```python
from build123d import *

# Parameters (mm, degrees)
BOSS_EXTRUDE1_DEPTH = 1


with BuildPart() as part:
    # Sketch1 → Revolve1 (revolve)
    with BuildSketch(Plane(origin=(0, 0, 0), x_dir=(1, 0, 0), z_dir=(0, 1, 0))):
        Polygon((0, 15.606821862), (12, 15.606821862), (12, -8.393178138), (9.5, -8.393178138), (9.5, -11.393178138), (1, -11.393178138), (1, -19.393178138), (0, -19.393178138), align=None)
    revolve(axis=Axis((0, 0, 19.393178138), (0, 0, -1)))

    # Sketch3 → Boss-Extrude1 (add, symmetric)
    with BuildSketch(Plane(origin=(0, 0, 0), x_dir=(1, 0, 0), z_dir=(0, 1, 0))):
        with BuildLine():
            Line((9.289467417, 15.291250115), (7.355842044, 18.774923355))
            ThreePointArc((7.355842044, 18.774923355), (7.60881313, 19.659037934), (8.492927709, 19.406066848))
            Line((8.492927709, 19.406066848), (10.426553083, 15.922393608))
            ThreePointArc((10.426553083, 15.922393608), (10.173581996, 15.038279029), (9.289467417, 15.291250115))
        make_face()
        with BuildLine():
            Line((-9.289467417, 15.291250115), (-7.355842044, 18.774923355))
            ThreePointArc((-7.355842044, 18.774923355), (-7.60881313, 19.659037934), (-8.492927709, 19.406066848))
            Line((-8.492927709, 19.406066848), (-10.426553083, 15.922393608))
            ThreePointArc((-10.426553083, 15.922393608), (-10.173581996, 15.038279029), (-9.289467417, 15.291250115))
        make_face()
    extrude(amount=BOSS_EXTRUDE1_DEPTH, both=True)


solid = part.part
```
Verification items for the finished model (mm, model axes). A direction names the side the tool comes from. Coordinates: 2 decimals unless noted, no trailing zeros. Loops run counter-clockwise (first coordinate to the right, second up) from the corner with the lowest first, then second, coordinate; pieces in that order, holes last. Notation, with made-up numbers: (78.25, 16) - (129.25, 16) arc R21 cw to (129.25, 50) - close; hole circle Ø11 at (-28.5, -8.75). An arc over 180 degrees is marked (long way). Answer as a JSON object with one key per item and string values.
(1) Cross-section at D-D, the plane y = -5.75. Record the boundary of the cut face in (x, z).
Response:
{"outline": "(-10.53, -15.61) - (10.53, -15.61) - (10.53, 8.39) - (7.56, 8.39) - (7.56, 11.39) - (-7.56, 11.39) - (-7.56, 8.39) - (-10.53, 8.39) - close"}
(2) Cross-section at C-C, the plane z = 13.5. Record the boundary of the cut face in (x, y), then the cut area to 3 significant figures.
Response:
{"outline": "circle Ø2 at (0, 0)", "area": "3.14 mm²"}
(3) Cross-section at B-B, the plane x = 0. Record the boundary of the cut face in (y, z), then the cut area to 3 significant figures.
Response:
{"outline": "(-12, -15.61) - (12, -15.61) - (12, 8.39) - (9.5, 8.39) - (9.5, 11.39) - (1, 11.39) - (1, 19.39) - (-1, 19.39) - (-1, 11.39) - (-9.5, 11.39) - (-9.5, 8.39) - (-12, 8.39) - close", "area": "649 mm²"}
(4) Access from +Z, -Z, +X, -X, +Y, -Y to the whole of each face (thin tool, end or side, straight path). Record for faces 1 (the flat face through (-9.446, 0.014, -17.689)), 2 (the flat face through (8.247, -0.014, -17.169)), 3 (the flat face through (-9, -1, -18)), 4 (the flat face through (-9, 1, -18)), 5 (the flat face through (9, -4, 8.393)).
Response:
{"face 1": "-Z, -X, +Y, -Y", "face 2": "+Y, -Y", "face 3": "-Z, +X, -X, -Y", "face 4": "-Z, +X, -X, +Y", "face 5": "+Z"}
(5) Go/stop test with flat-tipped pins: pin 1 Ø1.5 at (x, y) = (-2, -8.5) entering from -Z; pin 2 Ø1 at (y, z) = (-1, -14) entering from +X; pin 3 Ø6 at (y, z) = (0.5, -4.5) entering from -X; pin 4 Ø1.6 at (x, z) = (9.5, -18) entering from +Y. Record where each tip stops, or that it passes through.
Response:
{"pin 1": "stops at z = -15.61", "pin 2": "stops at x = 11.99", "pin 3": "stops at x = -12", "pin 4": "stops at y = 1"}
(6) Mould release check, pull along X, two halves, no side actions. Record for faces 6 (the flat face through (-8.247, 0.014, -17.169)), 7 (the flat face through (9, -1, -18)), 8 (the flat face through (9.446, -0.014, -17.689)): pulls with the +X half, pulls with the -X half, needs draft (parallel to the pull), parting line crosses it, or undercut.
Response:
{"face 6": "undercut", "face 7": "needs draft", "face 8": "pulls with the +X half"}
(7) Scan lines: line 1 along Z through (x, y) = (3.5, 8.5); line 2 along Z through (x, y) = (-1.5, -10); line 3 along Y through (x, z) = (6.25, 0). Record each from-to range of solid material in increasing order.
Response:
{"line 1": "z = -15.61 to 11.39", "line 2": "z = -15.61 to 8.39", "line 3": "y = -10.24 to 10.24"}
(8) Cross-section at A-A, the plane y = 0. Record the boundary of the cut face in (x, z).
Response:
{"outline": "(-12, -15.61) - (-10.51, -15.61) arc R0.65 ccw to (-10.43, -15.92) - (-8.49, -19.41) arc R0.65 ccw to (-7.36, -18.77) - (-9.11, -15.61) - (9.11, -15.61) - (7.36, -18.77) arc R0.65 ccw to (8.49, -19.41) - (10.43, -15.92) arc R0.65 ccw to (10.51, -15.61) - (12, -15.61) - (12, 8.39) - (9.5, 8.39) - (9.5, 11.39) - (1, 11.39) - (1, 19.39) - (-1, 19.39) - (-1, 11.39) - (-9.5, 11.39) - (-9.5, 8.39) - (-12, 8.39) - close"}
